```python
from build123d import *

# Parameters (mm, degrees)
U_SHAPE_DEPTH        = 100
FILLET_2_R           = 12
THICKNESS_T          = -10
SKETCH8_R            = 12.5
INNER_HOLE_DEPTH     = 122.757956619
TONGUE_DEPTH         = 10
SKETCH9_R            = 10
MOUNTING_HOLES_DEPTH = 197.53244007
FILLET1_R            = 5


with BuildPart() as part:
    # Sketch4 → "U" shape (new body)
    with BuildSketch(Plane.XY):
        with BuildLine():
            Line((-35, 0), (-35, -60))
            Line((-35, -60), (35, -60))
            Line((35, -60), (35, 0))
            ThreePointArc((35, 0), (0, 35), (-35, 0))
        make_face()
    extrude(amount=U_SHAPE_DEPTH)

    # Fillet 2
    fillet_2_edges = [part.edges().sort_by_distance(p)[0] for p in [
        (0, -60, 100),
        (0, -60, 0),
    ]]
    fillet(fillet_2_edges, radius=FILLET_2_R)

    # Thickness
    thickness_openings = [part.faces().sort_by_distance(p)[0] for p in [
        (35, -29.715655007, 50),
        (-35, -29.715655007, 50),
        (0, 35, 50),
    ]]
    offset(amount=THICKNESS_T, openings=thickness_openings, kind=Kind.INTERSECTION)

    # Sketch8 → Inner Hole (cut, through all)
    with BuildSketch(Plane.XY.offset(100)):
        Circle(SKETCH8_R)
    extrude(amount=-INNER_HOLE_DEPTH, mode=Mode.SUBTRACT)

    # Sketch7 → Tongue (add)
    with BuildSketch(Plane.XZ.offset(60)):
        with BuildLine():
            Line((35, 25), (115, 25))
            ThreePointArc((115, 25), (140, 50), (115, 75))
            Line((115, 75), (35, 75))
            Line((35, 75), (35, 25))
        make_face()
    extrude(amount=-TONGUE_DEPTH)

    # Sketch9 → Mounting Holes (cut, through all)
    with BuildSketch(Plane.XZ.offset(60)):
        with Locations((65, 50)):
            Circle(SKETCH9_R)
        with Locations((115, 50)):
            Circle(SKETCH9_R)
    extrude(amount=-MOUNTING_HOLES_DEPTH, mode=Mode.SUBTRACT)

    # Fillet1
    fillet1_edges = [part.edges().sort_by_distance(p)[0] for p in [
        (35, -55, 75),
        (35, -55, 25),
    ]]
    fillet(fillet1_edges, radius=FILLET1_R)


solid = part.part
```
Can you work these out from the model? Positions are in its coordinate system, mm. A direction names the side the tool comes from. Round coordinates to 2 decimals unless told otherwise and drop trailing zeros. Loops run counter-clockwise (first coordinate to the right, second up) from the corner with the lowest first, then second, coordinate; pieces in that order, holes last. Notation, with made-up numbers: M 16,10 L 42,10 A28 cw 42,30 Z; hole C -7,-39 d2. An arc over 180 degrees is marked long. Write item = value, one per line. Start each with the question number.
(1) Suppose I cut it at C-C on x = 0. Write out the boundary of the cut face in (y, z).
(2) Which directions (+Z, -Z, +X, -X, +Y, -Y) give clear straight access to the entire face, cutting with the end or side of a thin tool? Please do faces 5 (the face through (36, -55, 23)), 6 (the face through (0, -15, 10)), 7 (the face through (78, -55, 75)).
(3) Suppose I cut it at B-B on z = 50. Write out the boundary of the cut face in (x, y).
(4) If we mould it in two halves opening along X, with no side actions, what happens to faces 1 (the face through (112.83, -55.07, 40.24)), 2 (the face through (57, -55, 44)), 3 (the face through (35, -30, 8)), 4 (the face through (0.77, 34.99, 94.93))? For each: released by +X, released by -X, zero draft, split by the parting line, or undercut.
(5) I'm going to push flat-ended pins straight in: P1, Ø6, axis at y = -27, z = 8, coming from the +X side; P2, Ø8, axis at x = 92, y = -56.5, coming from the +Z side; P3, Ø23, axis at x = 65, z = 50, coming from the +Y side. Where does each tip first touch, or does it pass through?
(6) Suppose I cut it at D-D on y = -9. Write out the boundary of the cut face in (x, z), plus the area to 3 significant figures.
(7) I need wall thicknesses on line 1 along Z through (x, y) = (11, -19.5); line 2 along X through (y, z) = (-53.5, 58); line 3 along Z through (x, y) = (115, -57). Which ranges of each line are inside material? Lowest first, please.
(8) Suppose I cut it at A-A on x = 65. Write out the boundary of the cut face in (y, z).
Answer block:
q1.outline = M -60,12 A12 ccw -48,0 L -12.5,0 L -12.5,10 L -48,10 A2 cw -50,12 L -50,88 A2 cw -48,90 L -12.5,90 L -12.5,100 L -48,100 A12 ccw -60,88 Z; M 12.5,0 L 35,0 L 35,10 L 12.5,10 Z; M 12.5,90 L 35,90 L 35,100 L 12.5,100 Z
q2.face_5 = -Z, +X, +Y, -Y
q2.face_6 = +X, -X, +Y
q2.face_7 = +Z, +X, +Y, -Y
q3.outline = M -35,-60 L 55,-60 L 55,-50 L -35,-50 Z; M 75,-60 L 105,-60 L 105,-50 L 75,-50 Z; M 125,-60 L 140,-60 L 140,-50 L 125,-50 Z
q4.face_1 = undercut
q4.face_2 = undercut
q4.face_3 = released by +X
q4.face_4 = split by the parting line
q5.P1 = 35
q5.P2 = 75
q5.P3 = -50
q6.outline = M -35,0 L -8.67,0 L -8.67,10 L -35,10 Z; M -35,90 L -8.67,90 L -8.67,100 L -35,100 Z; M 8.67,0 L 35,0 L 35,10 L 8.67,10 Z; M 8.67,90 L 35,90 L 35,100 L 8.67,100 Z
q6.area = 1,050 mm²
q7.line_1 = 0 to 10, 90 to 100
q7.line_2 = -35 to 59, 71 to 109, 121 to 138.69
q7.line_3 = 25 to 40, 60 to 75
q8.outline = M -60,25 L -50,25 L -50,40 L -60,40 Z; M -60,60 L -50,60 L -50,75 L -60,75 Z
